Source: CAD feature listing. Evaluate the final solid. Frame: model axes, mm. Round coordinates to 2 decimals unless told otherwise and drop trailing zeros. Loops run counter-clockwise (first coordinate to the right, second up) from the corner with the lowest first, then second, coordinate; pieces in that order, holes last.
(1) Mould query, pull axis X, two halves, no side actions, for faces 1 (the conical face through (-0.78, 1.87, 5.23)), 2 (the flat face through (-2, -4, 0)), 3 (the cylindrical face through (-1.08, 4.88, 4.93)). Classes: pulls with the +X half, pulls with the -X half, needs draft (parallel to the pull), parting line crosses it, or undercut.
(2) Material intervals for probe 1 along Y at (x, z) = (0, 1.5); probe 2 along X at (y, z) = (2, 3.25); probe 3 along X at (y, z) = (3.25, 1), sorted ascending.
(3) First-contact query: pin 1 Ø1 at (y, z) = (4, 3) entering from +X; pin 2 Ø3 at (y, z) = (-2, 6) entering from +X; pin 3 Ø1 at (x, y) = (0.5, 1) entering from +Z. Flat tips, straight axial feed; report the tip coordinate or a pass-through.
(4) Section A-A, the plane z = 4.25. Return the cut outline in (x, y).
(5) Section B-B, the plane y = -4.5. Return the cut outline in (x, z).
(6) Section C-C, the plane z = 6.5. Return the cut outline in (x, y).
Autodesk Inventor part; units mm, degrees
ref_plane "YZ Plane" through (0, 0, 0) normal (1, 0, 0) x (0, 1, 0)
ref_plane "XZ Plane" through (0, 0, 0) normal (0, 1, 0) x (-1, 0, 0)
ref_plane "XY Plane" through (0, 0, 0) normal (0, 0, 1) x (1, 0, 0)
sketch "Sketch1" plane through (0, 0, 0) normal (0, 0, 1) x (1, 0, 0)
  circle A0 centre (0, 0) radius 5
  dimension "d0" = 10
extrude "Extrusion1" add sketch "Sketch1" along normal blind 10
sketch "Sketch2" plane through (0, 0, 0) normal (0, 0, -1) x (-1, 0, 0)
  point P0 (0, 0)
hole "Hole1" at (0, 0, 0) direction (0, 0, 1) diameter 1.25 end through all
chamfer "Chamfer1" distance 3.35 distance2 9 1 edges at (0, -0.625, 0) measured on face at (3.4917, -0.424, 0)
fillet "Fillet2" radius 1 2 edges at (0, -0.625, 10) (0, -0.625, 9)
properties part number "CableGuideInsert"
Output values:
1. face 1: undercut
1. face 2: needs draft
1. face 3: parting line crosses it
2. probe 1: y = -5 to -3.42, 3.42 to 5
2. probe 2: x = -4.58 to -1.91, 1.91 to 4.58
2. probe 3: x = -3.8 to -1.55, 1.55 to 3.8
3. pin 1: stops at x = 3.57
3. pin 2: stops at x = 4.97
3. pin 3: stops at z = 10
4. outline: circle Ø10 at (0, 0); hole circle Ø4.79 at (0, 0)
5. outline: (-2.18, 0) - (2.18, 0) - (2.18, 10) - (-2.18, 10) - close
6. outline: circle Ø10 at (0, 0); hole circle Ø3.11 at (0, 0)
